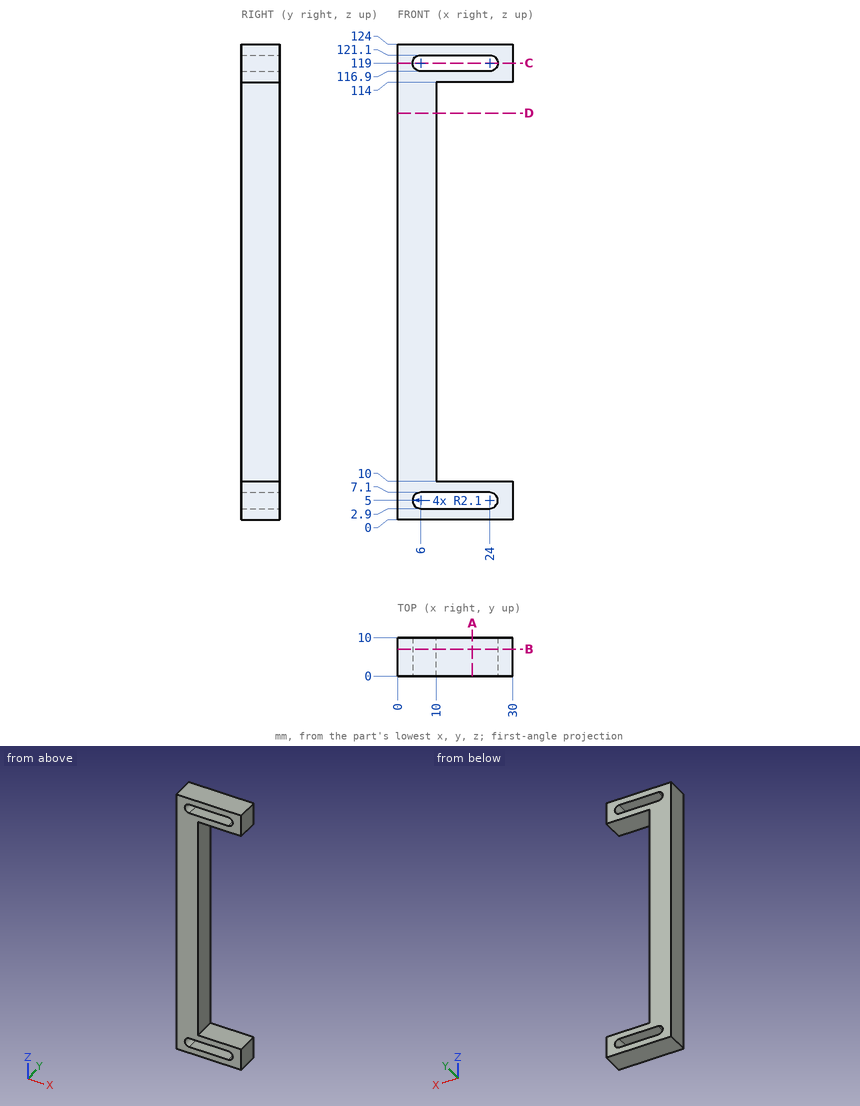
Could you check a few things on this drawing? It's one solid part, dimensions in mm from its lowest x, y, z. Give positions to 0.01 mm unless a question says otherwise; leave off trailing zeros. Write each loop counter-clockwise with the first axis right and the second up, starting at its lowest first coordinate (ties: lowest second). Pieces come first, ordered by that corner, then holes.
(1) If I drill on L1, parallel to Z at x = 22.5, y = 8; L2, parallel to Z at x = 7.5, y = 8.25; L3, parallel to Z at x = 27, y = 4, over which ranges is the centre line in solid material (lowest first)?
Output values:
L1: z = 0 to 2.9, 7.1 to 10, 114 to 116.9, 121.1 to 124
L2: z = 0 to 2.9, 7.1 to 116.9, 121.1 to 124
L3: z = 0 to 10, 114 to 124
(2) Imagine slicing it at A-A, the plane x = 19.5. Write out the boundary of the cut face in (y, z), and give its area (3 significant figures).
Output values:
outline: (0, 0) - (10, 0) - (10, 2.9) - (0, 2.9) - close; (0, 7.1) - (10, 7.1) - (10, 10) - (0, 10) - close; (0, 114) - (10, 114) - (10, 116.9) - (0, 116.9) - close; (0, 121.1) - (10, 121.1) - (10, 124) - (0, 124) - close
area: 116 mm2
(3) Imagine slicing it at D-D, the plane z = 106. Write out the boundary of the cut face in (x, y).
Output values:
outline: (0, 0) - (10, 0) - (10, 10) - (0, 10) - close
(4) Imagine slicing it at C-C, the plane z = 119. Write out the boundary of the cut face in (x, y), and give its area (3 significant figures).
Output values:
outline: (0, 0) - (3.9, 0) - (3.9, 10) - (0, 10) - close; (26.1, 0) - (30, 0) - (30, 10) - (26.1, 10) - close
area: 78.0 mm2
(5) Imagine slicing it at B-B, the plane y = 7. Write out the boundary of the cut face in (x, z).
Output values:
outline: (0, 0) - (30, 0) - (30, 10) - (10, 10) - (10, 114) - (30, 114) - (30, 124) - (0, 124) - close; hole (6, 2.9) - (24, 2.9) arc R2.1 ccw to (24, 7.1) - (6, 7.1) arc R2.1 ccw to start; hole (6, 116.9) - (24, 116.9) arc R2.1 ccw to (24, 121.1) - (6, 121.1) arc R2.1 ccw to start
